Work out the finished part from the listing and answer in its coordinate system (mm). Give positions to 0.01 mm unless a question says otherwise; leave off trailing zeros. Order: outer loops, then holes, each group sorted by start corner. A loop starts at its lowest first (then second) coordinate and runs counter-clockwise, first axis right, second up. Notation, with made-up numbers: (7.25, 7.5) - (26.25, 7.5) arc R14 ccw to (26.25, 23.5) - close; hole circle Ø11 at (18.25, 79). An arc over 180 degrees is marked (long way). Return JSON: item names as keys, results as strings. Group by question number.
Autodesk Inventor part; units mm, degrees
ref_plane "YZ Plane" through (0, 0, 0) normal (1, 0, 0) x (0, 1, 0)
ref_plane "XZ Plane" through (0, 0, 0) normal (0, 1, 0) x (-1, 0, 0)
ref_plane "XY Plane" through (0, 0, 0) normal (0, 0, 1) x (1, 0, 0)
sketch "Esboço1" plane through (0, 0, 0) normal (0, 1, 0) x (-1, 0, 0)
  line L0 (-42.5, 42.5) -> (42.5, 42.5)
  line L1 (42.5, 42.5) -> (42.5, -42.5)
  line L2 (42.5, -42.5) -> (-42.5, -42.5)
  line L3 (-42.5, -42.5) -> (-42.5, 42.5)
  line L4 (-42.5, 42.5) -> (42.5, -42.5) construction
  line L5 (42.5, 42.5) -> (-42.5, -42.5) construction
  point P0 (0, 0)
  dimension "d0" = 85
  dimension "d1" = 85
extrude "Extrusão1" add sketch "Esboço1" along normal blind 2
fillet "Arredondamento1" radius 2 4 edges at (42.5, 1, 42.5) (42.5, 1, -42.5) (-42.5, 1, 42.5) (-42.5, 1, -42.5)
sketch "Esboço2" plane through (0, 2, 0) normal (0, 1, 0) x (1, 0, 0)
  circle A0 centre (38.25, -38.25) radius 1.6
  line L0 (-40.5, -42.5) -> (40.5, -42.5)
  line L1 (42.5, -40.5) -> (42.5, 40.5)
  circle A1 centre (-38.25, 38.25) radius 1.6
  line L2 (-42.5, 40.5) -> (-42.5, -40.5)
  line L3 (40.5, 42.5) -> (-40.5, 42.5)
  point P0 (0, 0)
  dimension "d5" = 3.2
  dimension "d6" = 4.25
  dimension "d7" = 4.25
  dimension "d8" = 3.2
  dimension "d9" = 4.25
  dimension "d10" = 4.25
extrude "Extrusão2" cut sketch "Esboço2" against normal blind 2
properties part number "tampa caixa box"
1. Consider probe 1 along X at (y, z) = (1.4, -38.25); probe 2 along Z at (x, y) = (38.25, 1.35). Determine where each line is inside the solid, lowest interval first. Write a range as from..to.
2. The part is cut by section A-A (z = -38.25). Give the vertices of the cut face in (x, y).
3. This flat-tipped pin is pushed along its axis until it touches: pin 1 (2.5 mm diameter, centred on x = 38.25, z = 38.25, fed in from +Y). Where does it stop, or does it pass through?
4. The part is cut by section B-B (x = -38.25). Give the vertices of the cut face in (y, z), and give its area (3 significant figures).
5. Determine the mould class of faces 1 (the cylindrical face through (-37.51, 1.01, -36.83)), 2 (the cylindrical face through (41.93, 1.01, -41.9)), 3 (the flat face through (42.5, 1, -1)), 4 (the cylindrical face through (38.99, 1.01, 39.67)) for opening direction Z: released by +Z, released by -Z, zero draft, split by the parting line, or undercut.
Answers:
{
 "1": {"probe 1": "x = -42.5..-39.85, -36.65..42.5", "probe 2": "z = -42.5..36.65, 39.85..42.5"},
 "2": {"outline": "(-42.5, 0) - (-39.85, 0) - (-39.85, 2) - (-42.5, 2) - close; (-36.65, 0) - (42.5, 0) - (42.5, 2) - (-36.65, 2) - close"},
 "3": {"pin 1": "passes through"},
 "4": {"outline": "(0, -42.5) - (2, -42.5) - (2, -39.85) - (0, -39.85) - close; (0, -36.65) - (2, -36.65) - (2, 42.5) - (0, 42.5) - close", "area": "164 mm^2"},
 "5": {"face 1": "undercut", "face 2": "released by -Z", "face 3": "zero draft", "face 4": "undercut"}
}
